Source: CAD feature listing. Evaluate the final solid. Frame: model axes, mm. A direction names the side the tool comes from. Round coordinates to 2 decimals unless told otherwise and drop trailing zeros. Loops run counter-clockwise (first coordinate to the right, second up) from the corner with the lowest first, then second, coordinate; pieces in that order, holes last. Notation, with made-up numbers: (16.25, 83) - (49.25, 83) arc R25 ccw to (49.25, 106) - close; hole circle Ø6 at (60.5, 5). An arc over 180 degrees is marked (long way). Write item = value, one per line. Start each with the question number.
Autodesk Inventor part; units mm, degrees
ref_plane "YZ Plane" through (0, 0, 0) normal (1, 0, 0) x (0, 1, 0)
ref_plane "XZ Plane" through (0, 0, 0) normal (0, 1, 0) x (-1, 0, 0)
sketch "Sketch3" plane through (0, 0, 0) normal (0, 0, 1) x (1, 0, 0)
  line L0 (-12.7, -19.05) -> (12.7, -19.05)
  line L1 (12.7, -19.05) -> (12.7, 19.05)
  line L2 (12.7, 19.05) -> (-12.7, 19.05)
  line L3 (-12.7, 19.05) -> (-12.7, -19.05)
  line L4 (-12.7, -19.05) -> (12.7, 19.05) construction
  line L5 (12.7, -19.05) -> (-12.7, 19.05) construction
  point P0 (0, 0)
  dimension "d0" = 25.4
  dimension "d1" = 38.1
extrude "Extrusion1" add sketch "Sketch3" along normal mid plane 12.7
sketch "Sketch4" plane through (0, 0, 6.35) normal (0, 0, 1) x (1, 0, 0)
  circle A0 centre (0, 0) radius 2.667
  dimension "d4" = 5.334
extrude "Extrusion2" cut sketch "Sketch4" against normal through all
sketch "Sketch5" plane through (-12.7, -19.05, 6.35) normal (-1, 0, 0) x (0, 0, 1)
  line L0 (3.175, 6.35) -> (50.8, 6.35)
  line L1 (-12.7, 38.1) -> (-12.7, 0)
  line L2 (0, 0) -> (0, 38.1)
  line L3 (-12.7, 0) -> (0, 0)
  line L4 (0, 0) -> (0, 6.35)
  line L5 (0, 6.35) -> (-12.7, 6.35)
  line L6 (-12.7, 6.35) -> (-12.7, 0)
  point P0 (-6.35, 19.05)
  point P1 (-12.7, 6.35)
  dimension "d9" = 6.35
extrude "Extrusion3" cut sketch "Sketch5" against normal through all
sketch "Sketch8" plane through (-12.7, -12.7, -6.35) normal (-1, 0, 0) x (0, 0, 1)
  line L0 (-4.7625, 21.8398) -> (-4.7625, 13.2284)
  line L1 (12.7, 0) -> (12.7, 31.75)
  line L2 (12.7, 0) -> (-4.7625, 0)
  line L3 (-4.7625, 0) -> (-4.7625, 31.75)
  line L4 (-4.7625, 31.75) -> (12.7, 31.75)
  line L5 (12.7, 31.75) -> (12.7, 0)
  point P0 (6.35, 12.7)
  point P1 (-4.7625, 13.2284)
extrude "Extrusion5" add sketch "Sketch8" along normal blind 6.35
mirror "Mirror1" about plane through (0, 0, 0) normal (1, 0, 0) of "Extrusion5"
sketch "Sketch6" plane through (0, 0, 0) normal (0, 0, 1) x (1, 0, 0)
  circle A0 centre (0, 25.4) radius 15.367
  point P0 (0, 0)
  dimension "d10" = 25.4
  dimension "d13" = 30.734
extrude "cutOutForGuide" cut sketch "Sketch6" along normal mid plane 11.0998
sketch "Sketch9" plane through (0, 0, 6.35) normal (0, 0, 1) x (1, 0, 0)
  circle A0 centre (0, 0) radius 3.1242
  dimension "d16" = 6.2484
extrude "Extrusion6" cut sketch "Sketch9" against normal blind 9.525
split "Split1" plane through (0, 0, 0) removes the side toward (0, 0, 1)
properties part number "preventWireJumpingSingleSupportSliceB" material "PBT Plastic"
(1) Access query for faces 4 (the face through (12.7, 3, -9)), 5 (the face through (-16, 3, -11.112)), 6 (the face through (0.246, 10.035, -2.814)), 7 (the face through (2.98, 0.94, -1.57)). Directions: +Z, -Z, +X, -X, +Y, -Y. A direction counts if a zero-diameter tool reaches every point of the face in a straight line with its end or side. Return the directions, or none.
(2) Material intervals for line 1 along X through (y, z) = (-11, -8.75); line 2 along Y through (x, z) = (0, -4.55); line 3 along Y through (x, z) = (0, -0.9), sorted ascending. Write a range as from..to.
(3) Pin query (flat end, axial travel): P1, Ø10, axis at x = -0.5, y = -2, coming from the +Z side; P2, Ø7, axis at x = 1.5, y = 15.5, coming from the +Z side; P3, Ø5, axis at x = 0, y = 0, coming from the +Z side; P4, Ø8, axis at x = 3, y = 3.5, coming from the -Z side. Return the tip coordinate at first contact, or that it passes through.
(4) Cut plane C-C (z = -2.25). Output: boundary loops of the cut face in (x, y).
(5) Cut plane A-A (x = 0). Output: boundary loops of the cut face in (y, z) (3 decimals), and give its area (3 significant figures).
(6) Mould query, pull axis X, two halves, no side actions, for faces 1 (the face through (-5, -1, 0)), 2 (the face through (19.05, 3, -5)), 3 (the face through (0, 3, -6.35)). Classes: +X half, -X half, draft (parallel to the pull), parting line (faces both ways), or undercut.
(7) Cut plane D-D (z = -9.75). Output: boundary loops of the cut face in (x, y).
Solution:
q1.face_4 = -Z, +Y, -Y
q1.face_5 = -Z, +X, -X, +Y, -Y
q1.face_6 = +Z, +Y
q1.face_7 = +Z
q2.line_1 = -19.05..-12.7, 12.7..19.05
q2.line_2 = -12.7..-2.67, 2.67..10.03
q2.line_3 = -12.7..-3.12, 3.12..10.03
q3.P1 = 0
q3.P2 = -5.55
q3.P3 = through
q3.P4 = -6.35
q4.outline = (-19.05, -12.7) - (19.05, -12.7) - (19.05, 19.05) - (13.99, 19.05) arc R15.37 cw to (-13.99, 19.05) - (-19.05, 19.05) - close; hole circle Ø6.25 at (0, 0)
q5.outline = (-12.7, -6.35) - (-2.667, -6.35) - (-2.667, -3.175) - (-3.124, -3.175) - (-3.124, 0) - (-12.7, 0) - close; (2.667, -6.35) - (19.05, -6.35) - (19.05, -5.55) - (10.033, -5.55) - (10.033, 0) - (3.124, 0) - (3.124, -3.175) - (2.667, -3.175) - close
q5.area = 115 mm^2
q6.face_1 = draft
q6.face_2 = +X half
q6.face_3 = undercut
q7.outline = (-19.05, -12.7) - (-12.7, -12.7) - (-12.7, 19.05) - (-19.05, 19.05) - close; (12.7, -12.7) - (19.05, -12.7) - (19.05, 19.05) - (12.7, 19.05) - close
